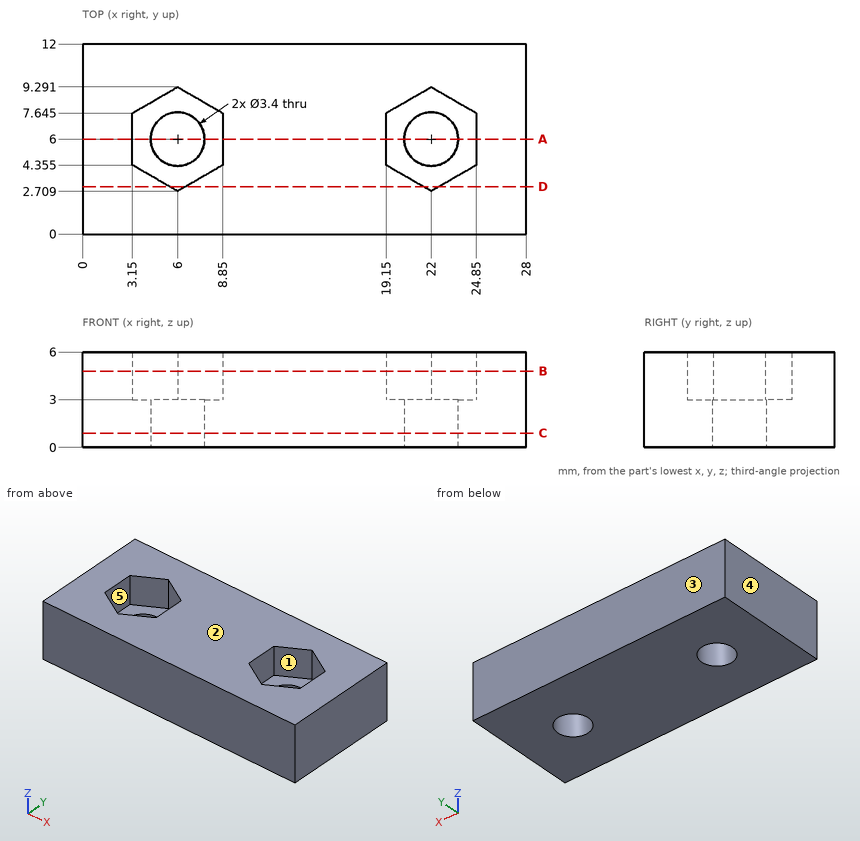
Study the drawing (mm; zero at the part's minimum x, y, z) and answer. A direction names the side the tool comes from. Give positions to 0.01 mm unless a question says otherwise; leave off trailing zeros. Order: outer loops, then holes, each group sorted by start corner. A loop starts at its lowest first (then second) coordinate and runs counter-clockwise, first axis right, second up.
1) Find section C-C on z = 0.9. Write down the section's boundary in (x, y), then the cut area to 3 significant figures.
Reported:
outline: (0, 0) - (28, 0) - (28, 12) - (0, 12) - close; hole circle Ø3.4 at (6, 6); hole circle Ø3.4 at (22, 6)
area: 318 mm2
2) For the marked faces 1 and 2, determine the directions among +Z, -Z, +X, -X, +Y, -Y from which every point of the face is accessible in a straight line to the end or side of a thin tool.
Reported:
face 1: +Z
face 2: +Z, +X, -X, +Y, -Y
3) Given P1, Ø1.5, axis at y = 5.5, z = 4.5, coming from the -X side; P2, Ø3, axis at x = 23, y = 5.5, coming from the +Z side, each flat-ended and moving along its own axis, determine where each tip first touches the part or whether it passes through.
Reported:
P1: stops at x = 0
P2: stops at z = 3
4) Find section D-D on y = 3. Write down the section's boundary in (x, z), then the cut area to 3 significant figures.
Reported:
outline: (0, 0) - (28, 0) - (28, 6) - (22.5, 6) - (22.5, 3) - (21.5, 3) - (21.5, 6) - (6.5, 6) - (6.5, 3) - (5.5, 3) - (5.5, 6) - (0, 6) - close
area: 162 mm2
5) Determine the mould class of the marked faces 3, 4 and 5 for opening direction X: pulls with the +X half, pulls with the -X half, needs draft (parallel to the pull), parting line crosses it, or undercut.
Reported:
face 3: needs draft
face 4: pulls with the -X half
face 5: undercut
6) Find section B-B on z = 4.8. Give the number of separate pieces and of enclosed holes in the cut face, then the cut area to 3 significant figures.
Reported:
separate pieces: 1
enclosed holes: 2
area: 280 mm2
7) Find section A-A on y = 6. Write down the section's boundary in (x, z).
Reported:
outline: (0, 0) - (4.3, 0) - (4.3, 3) - (3.15, 3) - (3.15, 6) - (0, 6) - close; (7.7, 0) - (20.3, 0) - (20.3, 3) - (19.15, 3) - (19.15, 6) - (8.85, 6) - (8.85, 3) - (7.7, 3) - close; (23.7, 0) - (28, 0) - (28, 6) - (24.85, 6) - (24.85, 3) - (23.7, 3) - close
8) Consider line 1 along X through (y, z) = (6, 1.05); line 2 along X through (y, z) = (7.5, 3.15); line 3 along Y through (x, z) = (22, 2.1). Determine where each line is inside the solid, lowest interval first.
Reported:
line 1: x = 0 to 4.3, 7.7 to 20.3, 23.7 to 28
line 2: x = 0 to 3.15, 8.85 to 19.15, 24.85 to 28
line 3: y = 0 to 4.3, 7.7 to 12
